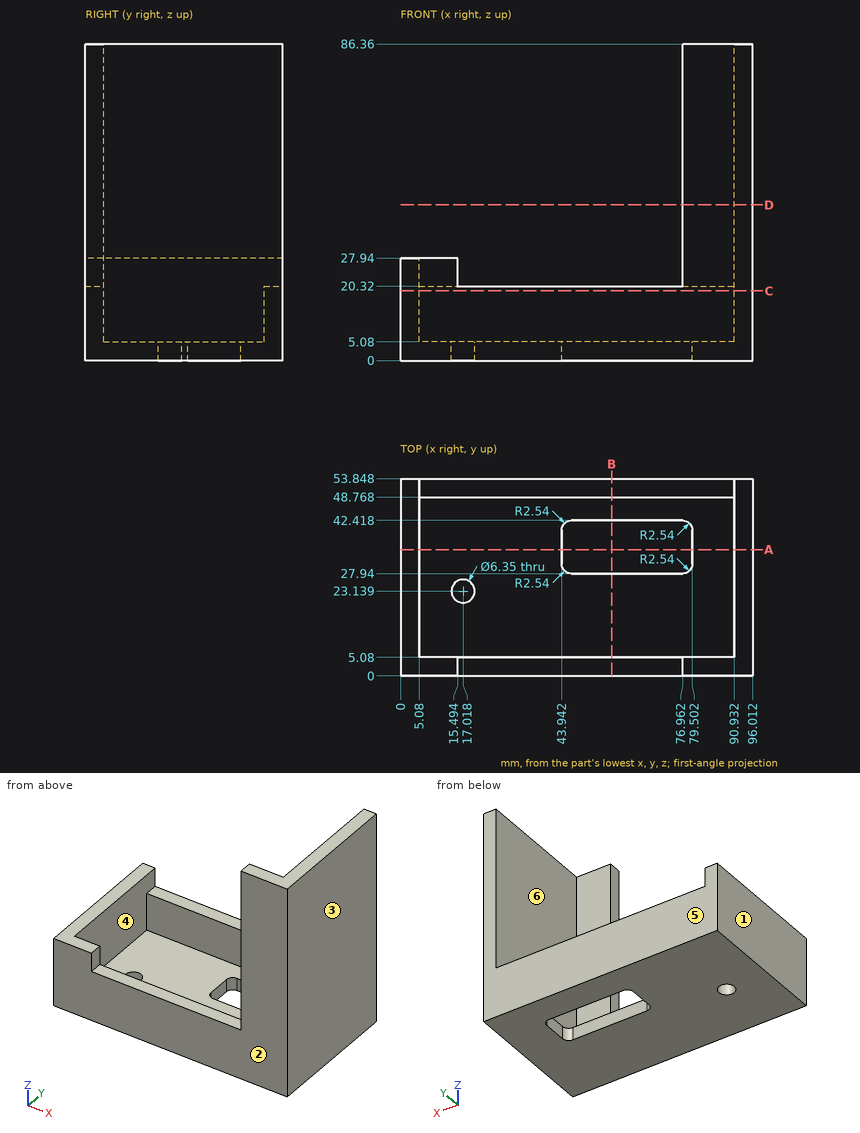
Source: three-view drawing plus pictorial views. Frame: mm from the lowest corner of the part. A direction names the side the tool comes from. Round coordinates to 2 decimals unless told otherwise and drop trailing zeros. Loops run counter-clockwise (first coordinate to the right, second up) from the corner with the lowest first, then second, coordinate; pieces in that order, holes last.
1. Contact query for flat-ended pins moving along their axis: pin 1 (4 mm diameter, centred on x = 40.5, y = 2.5, fed in from +Z); pin 2 (6 mm diameter, centred on x = 68.5, y = 7.5, fed in from -Z); pin 3 (10 mm diameter, centred on y = 19, z = 39.5, fed in from -X); pin 4 (2 mm diameter, centred on x = 78.5, z = 76.5, fed in from +Y). Output: stop coordinate, or through.
2. Mould query, pull axis X, two halves, no side actions, for the marked faces 1, 2, 3 and 4. Classes: released by +X, released by -X, zero draft, split by the parting line, or undercut.
3. Ray query, L1, parallel to X at y = 22, z = 13; L2, parallel to Y at x = 85, z = 40.5; L3, parallel to X at y = 25, z = 59. Return the intervals inside material, ascending.
4. Section query B-B on x = 57.5. Output: boundary loops of the cut face in (y, z), and give its area (3 significant figures).
5. Section query D-D on z = 42.5. Output: boundary loops of the cut face in (x, y).
6. Access query for the marked faces 5 and 6. Directions: +Z, -Z, +X, -X, +Y, -Y. A direction counts if a zero-diameter tool reaches every point of the face in a straight line with its end or side. Return the directions, or none.
7. Section query C-C on z = 19. Output: boundary loops of the cut face in (x, y).
8. Section query A-A on y = 34.5. Output: boundary loops of the cut face in (x, z), and give its area (3 significant figures).
Answers below:
1. pin 1: stops at z = 20.32
1. pin 2: stops at z = 0
1. pin 3: stops at x = 90.93
1. pin 4: stops at y = 5.08
2. face 1: released by -X
2. face 2: zero draft
2. face 3: released by +X
2. face 4: undercut
3. L1: x = 0 to 5.08, 90.93 to 96.01
3. L2: y = 0 to 5.08
3. L3: x = 90.93 to 96.01
4. outline: (0, 0) - (27.94, 0) - (27.94, 5.08) - (5.08, 5.08) - (5.08, 20.32) - (0, 20.32) - close; (42.42, 0) - (53.85, 0) - (53.85, 20.32) - (48.77, 20.32) - (48.77, 5.08) - (42.42, 5.08) - close
4. area: 355 mm2
5. outline: (76.96, 0) - (96.01, 0) - (96.01, 53.85) - (90.93, 53.85) - (90.93, 5.08) - (76.96, 5.08) - close
6. face 5: +Z, -Z, +X, -X, +Y
6. face 6: +Z
7. outline: (0, 0) - (96.01, 0) - (96.01, 53.85) - (0, 53.85) - close; hole (5.08, 5.08) - (90.93, 5.08) - (90.93, 48.77) - (5.08, 48.77) - close
8. outline: (0, 0) - (43.94, 0) - (43.94, 5.08) - (5.08, 5.08) - (5.08, 27.94) - (0, 27.94) - close; (79.5, 0) - (96.01, 0) - (96.01, 86.36) - (90.93, 86.36) - (90.93, 5.08) - (79.5, 5.08) - close
8. area: 836 mm2
